The model under review builds one solid part; all positions refer to its coordinate system, in mm. A direction names the side the tool comes from. Round coordinates to 2 decimals unless told otherwise and drop trailing zeros. Order: outer loops, then holes, each group sorted by start corner. A loop starts at its lowest first (then second) coordinate and runs counter-clockwise, first axis right, second up. Notation, with made-up numbers: M 27.5,63 L 45.5,63 A13 ccw 45.5,76 Z; hole C 66,49.25 d8. An arc over 180 degrees is marked long. Answer as a JSON object with one key per item and string values. Group by question number.
1. Add section A-A on x = 50.5. State the section outline as (y, z) points.
2. Add section D-D on z = 17.5. State the section outline as (x, y) points.
3. Mouldability with a two-part tool opening along X and no side actions: class faces 3 (the face through (90, 39, 0)), 4 (the face through (46, 39, 5)), 5 (the face through (0, 39, 0)) as released by +X, released by -X, zero draft, split by the parting line, or undercut.
4. Add section C-C on y = 46. State the section outline as (x, z) points, and give its area (3 significant figures).
5. To check wall thickness, follow probe 1 along Z at (x, y) = (62.5, 33); probe 2 along Z at (x, y) = (59.5, 52). State the ranges of each line that lie inside material, in increasing order. Write a range as [from, to].
6. Machinability: for faces 1 (the face through (44, 80, 0)), 2 (the face through (58.36, 43.8, 15.14)), which of the approach directions +Z, -Z, +X, -X, +Y, -Y give a long, thin tool a straight path to every point of the face, cutting with its end or side? Answer none if there is none.
7. Add section B-B on z = 12.5. State the section outline as (x, y) points, and give its area (3 significant figures).
```python
from build123d import *

# Parameters (mm, degrees)
SKETCH1_W     = 90
SKETCH1_H     = 80
BASE_DEPTH    = 25
SKETCH2_W     = 12.505871318
SKETCH2_H     = 18.704284341
POCKET_DEPTH  = 20
DRAFT10_ANGLE = 10
DRAFT20_ANGLE = 20
DRAFT30_ANGLE = 30
DRAFT40_ANGLE = 40


with BuildPart() as part:
    # Sketch1 → Base (new body, symmetric)
    with BuildSketch(Plane.XY):
        with Locations((45, 40)):
            Rectangle(SKETCH1_W, SKETCH1_H)
    extrude(amount=BASE_DEPTH, both=True)

    # Sketch2 → Pocket (cut)
    with BuildSketch(Plane.XY.offset(25)):
        with Locations((46.252935659, 39.352142171)):
            Rectangle(SKETCH2_W, SKETCH2_H)
    extrude(amount=-POCKET_DEPTH, mode=Mode.SUBTRACT)

    # Draft10
    draft10_faces = [part.faces().sort_by_distance(p)[0] for p in [
        (40, 39.35214217, 15),
    ]]
    draft(draft10_faces, Plane(origin=(40, 48.704284341, 5), x_dir=(1, 0, 0), z_dir=(0, 0, 1)), DRAFT10_ANGLE)

    # Draft20
    draft20_faces = [part.faces().sort_by_distance(p)[0] for p in [
        (45.334985554, 30, 15.411907484),
    ]]
    draft(draft20_faces, Plane(origin=(40, 48.704284341, 5), x_dir=(1, 0, 0), z_dir=(0, 0, 1)), DRAFT20_ANGLE)

    # Draft30
    draft30_faces = [part.faces().sort_by_distance(p)[0] for p in [
        (52.505871318, 37.433476694, 15.542980146),
    ]]
    draft(draft30_faces, Plane(origin=(40, 48.704284341, 5), x_dir=(1, 0, 0), z_dir=(0, 0, 1)), DRAFT30_ANGLE)

    # Draft40
    draft40_faces = [part.faces().sort_by_distance(p)[0] for p in [
        (48.509384653, 48.704284341, 16.253456142),
    ]]
    draft(draft40_faces, Plane(origin=(40, 48.704284341, 5), x_dir=(1, 0, 0), z_dir=(0, 0, 1)), DRAFT40_ANGLE)


solid = part.part
```
Recorded:
{
 "1": {"outline": "M 0,-25 L 80,-25 L 80,25 L 65.49,25 L 48.7,5 L 30,5 L 22.72,25 L 0,25 Z"},
 "2": {"outline": "M 0,0 L 90,0 L 90,80 L 0,80 Z; hole M 37.8,25.45 L 59.72,25.45 L 59.72,59.19 L 37.8,59.19 Z"},
 "3": {"face 3": "released by +X", "face 4": "undercut", "face 5": "released by -X"},
 "4": {"outline": "M 0,-25 L 90,-25 L 90,25 L 64.05,25 L 52.51,5 L 40,5 L 36.47,25 L 0,25 Z", "area": "4,100 mm²"},
 "5": {"probe 1": "z = [-25, 22.31]", "probe 2": "z = [-25, 17.11]"},
 "6": {"face 1": "+Z, -Z, +X, -X, +Y", "face 2": "+Z"},
 "7": {"outline": "M 0,0 L 90,0 L 90,80 L 0,80 Z; hole M 38.68,27.27 L 56.84,27.27 L 56.84,55 L 38.68,55 Z", "area": "6,700 mm²"}
}
